The listing builds one solid part. Answer for the finished solid, in the listing's coordinates (mm). Face numbers are marked on the shaded views. A direction names the side the tool comes from. Coordinates: 2 decimals unless noted, no trailing zeros. Write each loop counter-clockwise with the first axis right and the second up, starting at its lowest first coordinate (ties: lowest second). Pieces come first, ordered by that corner, then holes.
(1) For a pull along Z with two mould halves and no side action, classify the marked faces 1, 2 and 3 as +Z half, -Z half, draft (parallel to the pull), parting line (faces both ways), or undercut.
(2) The part is cut by section D-D on y = 19.5. Determine the outline of the cut face in (x, z).
(3) The part is cut by section C-C on x = -46. Determine the outline of the cut face in (y, z), plus the area to 3 significant figures.
(4) Which of the six approach directions +Z, -Z, +X, -X, +Y, -Y give full straight-line access (tool end or side, diameter ignored) to the marked faces 4 and 5?
(5) The part is cut by section A-A on y = -12. Determine the outline of the cut face in (x, z).
(6) Straight lines are drawn through the part: line 1 (Z direction, x = -38, y = 9.5); line 2 (X direction, y = 0, z = 11.8); line 3 (Y direction, x = -55, z = 12.15). For each, find the intervals that lie inside material, in ascending order.
(7) The part is cut by section B-B on z = 16.5. Determine the outline of the cut face in (x, y), plus the area to 3 significant figures.
(8) Given P1, Ø2.5, axis at x = -54.5, y = -1, coming from the -Z side; P2, Ø5, axis at x = -54.5, z = 15, coming from the -Y side; P3, Ø4, axis at x = -57, z = 18, coming from the -Y side, each flat-ended and moving along its own axis, determine where each tip first touches the part or whether it passes through.
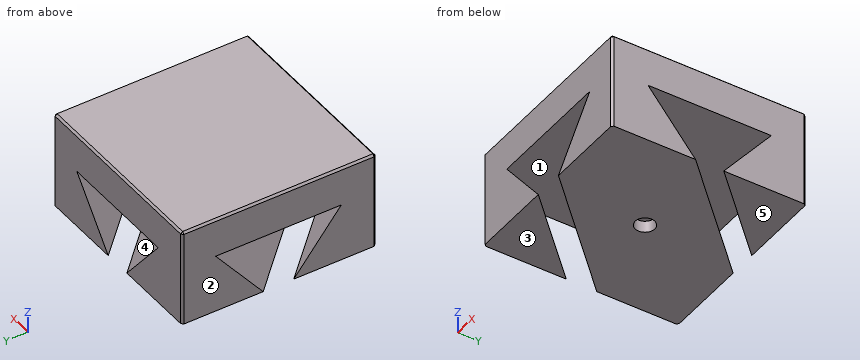
from build123d import *

# Parameters (mm, degrees)
F0_W      = 50
F0_H      = 50
F1_DEPTH  = 25
F4_DEPTH  = 70.7116781187
F5_W      = 50
F5_H      = 50
F6_DEPTH  = 25
F9_SIZE   = 0.5
F11_R     = 2.5
F12_DEPTH = 3


with BuildPart() as f1:
    # F0 (on Top) → F1 (new body)
    with BuildSketch(Plane.XY):
        Rectangle(F0_W, F0_H)
    extrude(amount=F1_DEPTH)

    # F3 (on face) → F4 (cut, through all)
    with BuildSketch(Plane(origin=(25, -25, 0), x_dir=(-0.7071067812, -0.7071067812, 0), z_dir=(-0.7071067812, 0.7071067812, 0))):
        Polygon((35.3553390593, 25), (29.0155930972, 25), (20.3553390593, 10), (35.3553390593, 10), align=None)
        Polygon((-20.3553390593, 10), (-29.0155930972, 25), (-35.3553390593, 25), (-35.3553390593, 10), align=None)
        Polygon((6.1227716358, 25), (0, 25), (-6.5567202885, 25), (-15.2169743263, 10), (14.7830256737, 10), align=None)
    extrude(amount=F4_DEPTH, mode=Mode.SUBTRACT)


with BuildPart() as f6:
    # F5 (on face) → F6 (new body)
    with BuildSketch(Plane.XY.offset(10)):
        Rectangle(F5_W, F5_H)
    extrude(amount=F6_DEPTH)

    # F7: cut F1
    add(f1.part, mode=Mode.SUBTRACT)


with BuildPart() as f6_1:
    # F8: moved
    add(f6.part.moved(Location((-55, 0, 0))))

    # F9
    f9_edges = [f6_1.edges().sort_by_distance(p)[0] for p in [
        (-80, 25, 22.5),
        (-80, -25, 22.5),
        (-30, 25, 22.5),
        (-30, -25, 22.5),
        (-30, 0, 35),
        (-55, 25, 35),
        (-80, 0, 35),
        (-55, -25, 35),
    ]]
    chamfer(f9_edges, length=F9_SIZE)

    # F11 (on face) → F12 (cut)
    with BuildSketch(Plane(origin=(0, 0, 10), x_dir=(1, 0, 0), z_dir=(0, 0, -1))):
        with Locations((-55, 0)):
            Circle(F11_R)
    extrude(amount=-F12_DEPTH, mode=Mode.SUBTRACT)


solid = f6_1.part
Model answer:
1. face 1: undercut
1. face 2: draft
1. face 3: -Z half
2. outline: (-80, 10) - (-52.98, 10) - (-65.23, 25) - (-33.47, 25) - (-45.71, 10) - (-30, 10) - (-30, 34.5) - (-30.5, 35) - (-79.5, 35) - (-80, 34.5) - close
3. outline: (-25, 10) - (12.52, 10) - (0.27, 25) - (25, 25) - (25, 34.5) - (24.5, 35) - (-24.5, 35) - (-25, 34.5) - (-25, 25) - (-17.66, 25) - (-25, 16.01) - close; (19.79, 10) - (25, 10) - (25, 16.38) - close
3. area: 954 mm2
4. face 4: none
4. face 5: -Z, +X, -X, +Y, -Y
5. outline: (-80, 10) - (-71.79, 10) - (-80, 20.06) - close; (-80, 25) - (-51.66, 25) - (-63.91, 10) - (-30, 10) - (-30, 20.43) - (-33.73, 25) - (-30, 25) - (-30, 34.5) - (-30.5, 35) - (-79.5, 35) - (-80, 34.5) - close
6. line 1: z = 25 to 35
6. line 2: x = -74.44 to -57.5, -52.5 to -34.95
6. line 3: y = -19.15 to -2.5, 2.5 to 19.76
7. outline: (-80, -24.5) - (-79.5, -25) - (-64.09, -25) - (-80, -9.09) - close; (-80, 9.4) - (-45.6, -25) - (-30.5, -25) - (-30, -24.5) - (-30, -8.79) - (-63.79, 25) - (-79.5, 25) - (-80, 24.5) - close; (-45.91, 25) - (-30, 9.09) - (-30, 24.5) - (-30.5, 25) - close
7. area: 1,590 mm2
8. P1: stops at z = 13
8. P2: stops at y = -20.55
8. P3: stops at y = -14.96
